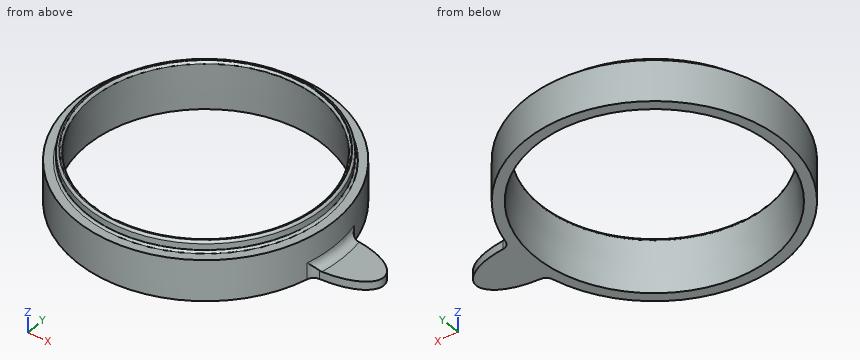
```python
from build123d import *

# Parameters (mm, degrees)
SKETCH_R        = 62.5
PAD_DEPTH       = 20
SKETCH001_R     = 57.5
POCKET_DEPTH    = 20.001
SKETCH002_R     = 57.5
PAD001_DEPTH    = 25
SKETCH003_R     = 55
POCKET001_DEPTH = 25.001
FILLET_R        = 1
PAD002_DEPTH    = 4
FILLET001_R     = 4


with BuildPart() as part:
    # Sketch → Pad (new body)
    with BuildSketch(Plane.XY):
        Circle(SKETCH_R)
    extrude(amount=PAD_DEPTH)

    # Sketch001 (on Face3 of Pad) → Pocket (cut, through all)
    with BuildSketch(Plane.XY.offset(20)):
        Circle(SKETCH001_R)
    extrude(amount=-POCKET_DEPTH, mode=Mode.SUBTRACT)

    # Sketch002 → Pad001 (join)
    with BuildSketch(Plane.XY):
        Circle(SKETCH002_R)
    extrude(amount=PAD001_DEPTH)

    # Sketch003 (on Face6 of Pad001) → Pocket001 (cut, through all)
    with BuildSketch(Plane.XY.offset(25)):
        Circle(SKETCH003_R)
    extrude(amount=-POCKET001_DEPTH, mode=Mode.SUBTRACT)

    # Sketch004 → Groove (revolve, cut)
    with BuildSketch(Plane.XZ):
        Polygon((-57.5, 0), (-55, 0), (-55, 25), align=None)
    revolve(axis=Axis((0, 0, 0), (0, 0, 1)), mode=Mode.SUBTRACT)

    # Fillet
    fillet_edges = [part.edges().sort_by_distance(p)[0] for p in [
        (-57.5, 0, 25),
        (0, 55, 25),
        (0, -55, 25),
        (-57.5, 0, 20),
        (57.5, 0, 22.5),
    ]]
    fillet(fillet_edges, radius=FILLET_R)

    # Sketch005 → Pad002 (join)
    with BuildSketch(Plane.XY):
        with BuildLine():
            add(Edge.make_bspline(
                [(61.361633, -11.874342), (86.361633, -11.874342), (86.361633, 0), (86.361633, 11.874342), (61.361633, 11.874342)],
                knots=[4.712389, 4.712389, 4.712389, 6.283185, 6.283185, 7.853982, 7.853982, 7.853982], degree=2, weights=[1, 0.707107, 1, 0.707107, 1]))
            ThreePointArc((61.361633, 11.874342), (62.5, 0), (61.361633, -11.874342))
        make_face()
    extrude(amount=PAD002_DEPTH)

    # Fillet001
    fillet001_edges = [part.edges().sort_by_distance(p)[0] for p in [
        (61.361633, -11.874342, 2),
        (62.214757, -5.964392, 4),
        (62.214757, 5.964392, 4),
        (61.361633, 11.874342, 2),
    ]]
    fillet(fillet001_edges, radius=FILLET001_R)


solid = part.part
```
Read the model definition and answer for the solid it produces. Units are mm, in the model's axes. Give positions to 0.01 mm unless a question says otherwise; leave off trailing zeros. Write each loop counter-clockwise with the first axis right and the second up, starting at its lowest first coordinate (ties: lowest second). Pieces come first, ordered by that corner, then holes. Notation, with made-up numbers: (-34.75, -3) - (12.25, -3) arc R21 ccw to (12.25, 28) - close; hole circle Ø3 at (-7.75, 89). An arc over 180 degrees is marked (long way). Write item = value, one per line. Start each with the question number.
Item 1: Each of these flat-tipped pins is pushed along its axis until it touches: P1, Ø12, axis at y = 28.5, z = 10, coming from the -X side; P2, Ø1.5, axis at x = 65, z = 9.5, coming from the +Y side; P3, Ø23, axis at x = 72, y = 1, coming from the +Z side; P4, Ø6, axis at x = 14, z = 11.5, coming from the -Y side. Where does it stop, or does it pass through?
Item 2: Find the intervals of material crossed by probe 1 along Y at (x, z) = (-22.5, 21.75); probe 2 along Y at (x, z) = (46, 21.5); probe 3 along X at (y, z) = (26, 13.5), in increasing order. Write a range as [from, to].
Item 3: Find section B-B (z = 12). Give the vertices of the cut face in (x, y), then the cut area to 3 significant figures.
Item 4: Find section A-A (x = 0). Give the vertices of the cut face in (y, z), then the cut area to 3 significant figures.
Response:
q1.P1 = -58.31
q1.P2 = through
q1.P3 = 20
q1.P4 = -61.52
q2.probe_1 = [-52.92, -50.54], [50.54, 52.92]
q2.probe_2 = [-34.5, -30.78], [30.78, 34.5]
q2.probe_3 = [-56.84, -49.77], [49.77, 56.84]
q3.outline = circle Ø125 at (0, 0); hole circle Ø112.6 at (0, 0)
q3.area = 2,310 mm²
q4.outline = (-62.5, 0) - (-57.5, 0) - (-55.11, 23.9) arc R1 ccw to (-56.1, 25) - (-56.5, 25) arc R1 ccw to (-57.5, 24) - (-57.5, 21) arc R1 cw to (-58.5, 20) - (-62.5, 20) - close; (55.11, 23.9) - (57.5, 0) - (62.5, 0) - (62.5, 20) - (58.5, 20) arc R1 cw to (57.5, 21) - (57.5, 24) arc R1 ccw to (56.5, 25) - (56.1, 25) arc R1 ccw to start
q4.area = 262 mm²
